```python
from build123d import *

# Parameters (mm, degrees)
F0_W     = 111.7000012129
F0_H     = 26.4022397026
F1_DEPTH = 3
F2_DEPTH = 4


with BuildPart() as f1:
    # F0 (on Top) → F1 (new body)
    with BuildSketch(Plane.XY):
        Polygon((-53.1748010613, 0), (-65.0856580366, 0), (-65.8500006691, -1.1812567956), (-65.8500006691, -103.9500006691), (65.8500006691, -103.9500006691), (65.8500006691, -1.1812567956), (65.0856580366, 0), (53.1748010613, 0), (55.8500006065, -4.1343992971), (55.8500006065, -67.5477609038), (55.8500006065, -93.9500006065), (-55.8500006065, -93.9500006065), (-55.8500006065, -67.5477609038), (-55.8500006065, -4.1343992971), align=None)
        with Locations((0, -80.7488807551)):
            Rectangle(F0_W, F0_H)
        Polygon((0, 82.1792380038), (-25.8823529412, 42.1792380038), (25.8823529412, 42.1792380038), align=None)
        Polygon((0, 100.5869260566), (-65.0856580366, 0), (-53.1748010613, 0), (-25.8823529412, 42.1792380038), (0, 82.1792380038), (25.8823529412, 42.1792380038), (53.1748010613, 0), (65.0856580366, 0), align=None)
    extrude(amount=F1_DEPTH)

    # F0 (on Top) → F2 (join)
    with BuildSketch(Plane.XY):
        Polygon((-69.85, 0), (-69.85, -107.95), (69.85, -107.95), (69.85, 0), (65.0856580366, 0), (65.8500006691, -1.1812567956), (65.8500006691, -103.9500006691), (-65.8500006691, -103.9500006691), (-65.8500006691, -1.1812567956), (-65.0856580366, 0), align=None)
        Polygon((0, 107.95), (-69.85, 0), (-65.0856580366, 0), (0, 100.5869260566), (65.0856580366, 0), (69.85, 0), align=None)
    extrude(amount=F2_DEPTH)


solid = f1.part
```
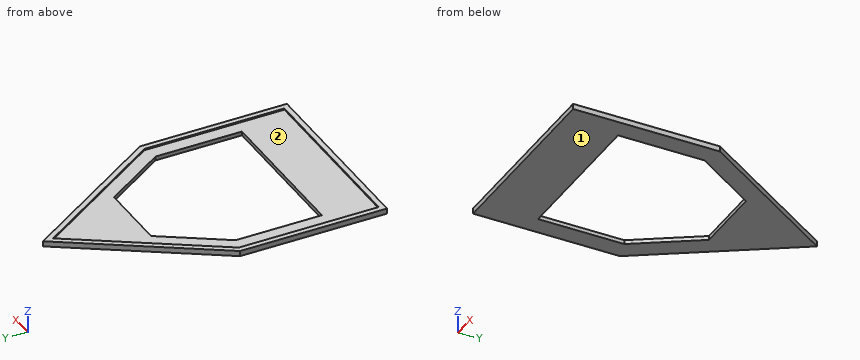
Part model, mm, in its own coordinate system. Face numbers are marked on the shaded views. Round coordinates to 2 decimals unless told otherwise and drop trailing zeros. Write each loop counter-clockwise with the first axis right and the second up, starting at its lowest first coordinate (ties: lowest second). Pieces come first, ordered by that corner, then holes. Notation, with made-up numbers: (73, 83) -> (117, 83) arc R28 ccw to (117, 114) -> close; hole circle Ø2 at (29.25, -10). An arc over 180 degrees is marked (long way). Return JSON: item names as keys, results as strings. Group by question number.
Q1. Saw through at B-B on y = -33.5. Write the cut outline in (x, z).
Q2. Saw through at C-C on x = 17. Write the cut outline in (y, z).
Q3. Mould opens along X. For the marked faces 1 and 2 say: pulls with the +X half, pulls with the -X half, needs draft (parallel to the pull), parting line crosses it, or undercut.
Q4. Saw through at A-A on z = 1.4. Write the cut outline in (x, y).
Q5. Pin check, flat tips, straight feed: pin 1 (1 mm diameter, centred on x = -1.5, y = -76.5, fed in from +Z); pin 2 (10 mm diameter, centred on x = -50, y = 43.5, fed in from -Z). Stop position of each tip, or through.
Q6. Probe L1, parallel to X at y = -44.5, z = 2.85; L2, parallel to X at y = -45, z = 3.05; L3, parallel to Y at x = 44.5, z = 2.65. List the from-to ranges inside material, lowest first. Write a range as [from, to].
Q7. Saw through at D-D on y = -88.5. Write the cut outline in (x, z), plus the area to 3 significant figures.
Answer:
{
 "1": {"outline": "(-69.85, 0) -> (-55.85, 0) -> (-55.85, 3) -> (-65.85, 3) -> (-65.85, 4) -> (-69.85, 4) -> close; (55.85, 0) -> (69.85, 0) -> (69.85, 4) -> (65.85, 4) -> (65.85, 3) -> (55.85, 3) -> close"},
 "2": {"outline": "(-107.95, 0) -> (-67.55, 0) -> (-67.55, 3) -> (-103.95, 3) -> (-103.95, 4) -> (-107.95, 4) -> close; (42.18, 0) -> (81.68, 0) -> (81.68, 4) -> (74.31, 4) -> (74.31, 3) -> (42.18, 3) -> close"},
 "3": {"face 1": "needs draft", "face 2": "undercut"},
 "4": {"outline": "(-69.85, -107.95) -> (69.85, -107.95) -> (69.85, 0) -> (0, 107.95) -> (-69.85, 0) -> close; hole (-55.85, -67.55) -> (55.85, -67.55) -> (55.85, -4.13) -> (25.88, 42.18) -> (-25.88, 42.18) -> (-55.85, -4.13) -> close"},
 "5": {"pin 1": "z = 3", "pin 2": "through"},
 "6": {"L1": "[-69.85, -55.85], [55.85, 69.85]", "L2": "[-69.85, -65.85], [65.85, 69.85]", "L3": "[-107.95, -67.55], [13.41, 39.18]"},
 "7": {"outline": "(-69.85, 0) -> (69.85, 0) -> (69.85, 4) -> (65.85, 4) -> (65.85, 3) -> (-65.85, 3) -> (-65.85, 4) -> (-69.85, 4) -> close", "area": "427 mm2"}
}
